```python
from build123d import *

# Parameters (mm, degrees)
F0_R          = 22.5
F1_DEPTH      = 10
F1_DEPTH_BACK = 10
F2_W          = 15
F2_H          = 20
F3_DEPTH      = 7.5
F3_DEPTH_BACK = 7.5
F4_R          = 21.3
F5_DEPTH      = 9
F5_DEPTH_BACK = 9
F6_R          = 12.5
F7_DEPTH      = 3
F8_W          = 12.4
F8_H          = 25.2830533619
F8_W_2        = 28.802598262
F8_H_2        = 12.4
F9_DEPTH      = 6.2
F9_DEPTH_BACK = 6.2


with BuildPart() as f1:
    # F0 (on Top) → F1 (new body, two sides)
    with BuildSketch(Plane.XY) as f1_sk:
        Circle(F0_R)
    extrude(amount=F1_DEPTH)
    extrude(f1_sk.sketch, amount=-F1_DEPTH_BACK)

    # F2 (on Top) → F3 (join, two sides)
    with BuildSketch(Plane.XY) as f3_sk:
        with Locations((0, -22.5)):
            Rectangle(F2_W, F2_H)
    extrude(amount=F3_DEPTH)
    extrude(f3_sk.sketch, amount=-F3_DEPTH_BACK)

    # F4 (on Top) → F5 (cut, two sides)
    with BuildSketch(Plane.XY) as f5_sk:
        Circle(F4_R)
    extrude(amount=-F5_DEPTH, mode=Mode.SUBTRACT)
    extrude(f5_sk.sketch, amount=F5_DEPTH_BACK, mode=Mode.SUBTRACT)

    # F6 (on face) → F7 (cut)
    with BuildSketch(Plane.XY.offset(10)):
        Circle(F6_R)
    extrude(amount=-F7_DEPTH, mode=Mode.SUBTRACT)

    # F8 (on Top) → F9 (cut, two sides)
    with BuildSketch(Plane.XY) as f9_sk:
        with Locations((0, 18.841526681)):
            Rectangle(F8_W, F8_H)
        Polygon((6.2, 31.4830533619), (6.2, 6.2), (35.002598262, 6.2), align=None)
        with Locations((20.601299131, 0)):
            Rectangle(F8_W_2, F8_H_2)
    extrude(amount=-F9_DEPTH, mode=Mode.SUBTRACT)
    extrude(f9_sk.sketch, amount=F9_DEPTH_BACK, mode=Mode.SUBTRACT)


solid = f1.part
```
Design review of the part built by this model. Coordinates are the model's own, in mm. A direction names the side the tool comes from. Coordinates: 2 decimals unless noted, no trailing zeros. Write each loop counter-clockwise with the first axis right and the second up, starting at its lowest first coordinate (ties: lowest second). Pieces come first, ordered by that corner, then holes.
1) Mouldability with a two-part tool opening along Y and no side actions: class faces 5 (the flat face through (7.5, -27, 0)), 6 (the flat face through (9, -9, 9)), 7 (the flat face through (21, -6.2, 0)) as +Y half, -Y half, draft (parallel to the pull), parting line (faces both ways), or undercut.
2) Add section D-D (y = -24). Write out the cut boundary in (x, z), plus the area to 3 significant figures.
3) Add section C-C (z = -4). Write out the cut boundary in (x, y), plus the area to 3 significant figures.
4) Add section A-A (y = 0). Write out the cut boundary in (x, z).
5) Add section B-B (x = 0). Write out the cut boundary in (y, z).
6) To check wall thickness, follow L1, parallel to Y at x = 0, z = 9.35; L2, parallel to Z at x = -6.5, y = 14; L3, parallel to Z at x = 7, y = -10. State the ranges of each line that lie inside material, in increasing order.
7) Insertion check: pin 1 (12.5 mm diameter, centred on x = -3, y = -29.5, fed in from -Z); pin 2 (1 mm diameter, centred on x = 2, z = 6.5, fed in from +Y); pin 3 (13 mm diameter, centred on x = 1.5, y = 2.5, fed in from +Z). Each pin has a flat end and moves straight along its axis. Give the tip position at first contact, or say it passes through.
8) Machinability: for faces 1 (the flat face through (0, 0, -9)), 2 (the flat face through (-6.2, 21, 0)), 3 (the flat face through (-7.5, -27, 0)), 4 (the cylindrical face through (11.923, 3.755, 9.507)), which of the approach directions +Z, -Z, +X, -X, +Y, -Y give a long, thin tool a straight path to every point of the face, cutting with its end or side? Answer none if there is none.
Check result:
1. face 5: draft
1. face 6: undercut
1. face 7: +Y half
2. outline: (-7.5, -7.5) - (7.5, -7.5) - (7.5, 7.5) - (-7.5, 7.5) - close
2. area: 225 mm2
3. outline: (-7.5, -32.5) - (7.5, -32.5) - (7.5, -21.21) arc R22.5 ccw to (21.63, -6.2) - (20.38, -6.2) arc R21.3 cw (long way) to (-6.2, 20.38) - (-6.2, 21.63) arc R22.5 ccw to (-7.5, -21.21) - close
3. area: 265 mm2
4. outline: (-22.5, -10) - (22.5, -10) - (22.5, -6.2) - (21.3, -6.2) - (21.3, -9) - (-21.3, -9) - (-21.3, 9) - (-12.5, 9) - (-12.5, 10) - (-22.5, 10) - close; (12.5, 9) - (21.3, 9) - (21.3, 6.2) - (22.5, 6.2) - (22.5, 10) - (12.5, 10) - close
5. outline: (-32.5, -7.5) - (-22.5, -7.5) - (-22.5, -10) - (22.5, -10) - (22.5, -6.2) - (21.3, -6.2) - (21.3, -9) - (-21.3, -9) - (-21.3, 9) - (-12.5, 9) - (-12.5, 10) - (-22.5, 10) - (-22.5, 7.5) - (-32.5, 7.5) - close; (12.5, 9) - (21.3, 9) - (21.3, 6.2) - (22.5, 6.2) - (22.5, 10) - (12.5, 10) - close
6. L1: y = -22.5 to -12.5, 12.5 to 22.5
6. L2: z = -10 to -9, 9 to 10
6. L3: z = -10 to -9
7. pin 1: stops at z = -7.5
7. pin 2: stops at y = 22.45
7. pin 3: stops at z = -9
8. face 1: none
8. face 2: +X, +Y
8. face 3: +Z, -Z, -X, -Y
8. face 4: +Z
